Autodesk Fusion 360 part; units mm, degrees
sketch "Boceto1" plane through (0, 0, 0) normal (0, 0, 1) x (1, 0, 0)
  line L0 (-67.5, 45) -> (67.5, 45)
  line L1 (67.5, 45) -> (67.5, -45)
  line L2 (67.5, -45) -> (-67.5, -45)
  line L3 (-67.5, -45) -> (-67.5, 45)
  line L4 (-67.5, 45) -> (67.5, -45) construction
  line L5 (67.5, 45) -> (-67.5, -45) construction
  dimension "d1" = 135
  dimension "d2" = 90
extrude "Extruir1" add sketch "Boceto1" along normal blind 4
sketch "Boceto2" plane through (0, 0, 4) normal (0, 0, 1) x (-1, 0, 0)
  line L0 (67.5, 45) -> (-67.5, 45)
  line L1 (-67.5, 45) -> (-67.5, -45)
  line L2 (-67.5, -45) -> (67.5, -45)
  line L3 (67.5, -45) -> (67.5, 45)
  line L4 (67.5, -45) -> (67.5, -40)
  line L5 (67.5, -40) -> (62.5, -40)
  line L6 (67.5, 45) -> (62.5, 45)
  line L7 (62.5, 45) -> (62.5, 40)
  line L8 (-67.5, -45) -> (-62.5, -45)
  line L9 (-62.5, -45) -> (-62.5, -40)
  line L10 (-67.5, 45) -> (-67.5, 40)
  line L11 (-67.5, 40) -> (-62.5, 40)
  circle A0 centre (62.5, -40) radius 2
  circle A1 centre (62.5, 40) radius 2
  circle A2 centre (-62.5, -40) radius 2
  circle A3 centre (-62.5, 40) radius 2
  dimension "d5" = 5
  dimension "d6" = 5
  dimension "d7" = 135
  dimension "d8" = 90
  dimension "d9" = 5
  dimension "d10" = 5
  dimension "d11" = 5
  dimension "d12" = 5
  dimension "d13" = 5
  dimension "d14" = 5
  dimension "d15" = 4
  dimension "d16" = 4
  dimension "d17" = 4
  dimension "d18" = 4
extrude "Extruir2" cut sketch "Boceto2" against normal blind 4 contours A1 | A3 | A2 | A0
fillet "Empalme1" radius 5 4 edges at (-67.5, -45, 2) (67.5, -45, 2) (67.5, 45, 2) (-67.5, 45, 2)
sketch "Boceto3" plane through (0, 0, 4) normal (0, 0, 1) x (-1, 0, 0)
  circle A0 centre (62.5, 40) radius 2
  circle A1 centre (-62.5, -40) radius 2
  circle A2 centre (62.5, -40) radius 2
  circle A3 centre (-62.5, 40) radius 2
  arc A4 (62.5, -45) -> (67.5, -40) centre (62.5, -40) ccw
  line L0 (67.5, -40) -> (67.5, 40)
  arc A5 (67.5, 40) -> (62.5, 45) centre (62.5, 40) ccw
  line L1 (62.5, 45) -> (-62.5, 45)
  arc A6 (-62.5, 45) -> (-67.5, 40) centre (-62.5, 40) ccw
  line L2 (-67.5, 40) -> (-67.5, -40)
  arc A7 (-67.5, -40) -> (-62.5, -45) centre (-62.5, -40) ccw
  line L3 (-62.5, -45) -> (62.5, -45)
  line L4 (-67.5, 0) -> (-46, 0)
  circle A8 centre (-46, 0) radius 4
  circle A9 centre (-46, 0) radius 7
  line L5 (-46, 0) -> (-46, -7) construction
  line L6 (-46, 0) -> (-39, 0) construction
  line L7 (-46, 0) -> (-46, 7) construction
  line L8 (-46, 0) -> (-53, 0) construction
  circle A10 centre (-46, -7) radius 1.5
  circle A11 centre (-39, 0) radius 1.5
  circle A12 centre (-46, 7) radius 1.5
  circle A13 centre (-53, 0) radius 1.5
  dimension "d23" = 21.5
  dimension "d24" = 8
  dimension "d25" = 14
  dimension "d26" = 3
  dimension "d27" = 3
  dimension "d28" = 3
  dimension "d29" = 3
extrude "Extruir3" cut sketch "Boceto3" against normal blind 4 contours L4 A9 A13 | L4 A9 A13 | L4 A9 A13 | L4 A9 A13 | A8 | A9 A12 | A9 A12 | A9 A10 | A9 A10 | A9 A11 | A9 A11
mirror "Simetría1" about plane through (0, 0, 0) normal (1, 0, 0) of "Extruir3"
sketch "Boceto4" plane through (0, 0, 4) normal (0, 0, 1) x (-1, 0, 0)
  circle A0 centre (46, 7) radius 1.5
  circle A1 centre (46, -7) radius 1.5
  circle A2 centre (39, 0) radius 1.5
  circle A3 centre (53, 0) radius 1.5
  circle A4 centre (46, 0) radius 4
  arc A5 (62.5, -45) -> (67.5, -40) centre (62.5, -40) ccw
  line L0 (67.5, -40) -> (67.5, 40)
  arc A6 (67.5, 40) -> (62.5, 45) centre (62.5, 40) ccw
  line L1 (62.5, 45) -> (-62.5, 45)
  arc A7 (-62.5, 45) -> (-67.5, 40) centre (-62.5, 40) ccw
  line L2 (-67.5, 40) -> (-67.5, -40)
  arc A8 (-67.5, -40) -> (-62.5, -45) centre (-62.5, -40) ccw
  line L3 (-62.5, -45) -> (62.5, -45)
  circle A9 centre (-62.5, 40) radius 2
  circle A10 centre (62.5, -40) radius 2
  circle A11 centre (-62.5, -40) radius 2
  circle A12 centre (62.5, 40) radius 2
  circle A13 centre (-46, 7) radius 1.5
  circle A14 centre (-46, -7) radius 1.5
  circle A15 centre (-53, 0) radius 1.5
  circle A16 centre (-39, 0) radius 1.5
  circle A17 centre (-46, 0) radius 4
  line L4 (0, 35) -> (0, -35)
  line L5 (-20, -35) -> (20, -35)
  line L6 (-20, 35) -> (20, 35)
  line L7 (20, -30) -> (-20, -30)
  arc A18 (-20, -30) -> (-20, -40) centre (-20, -35) ccw
  line L8 (-20, -40) -> (20, -40)
  arc A19 (20, -40) -> (20, -30) centre (20, -35) ccw
  line L9 (20, -35) -> (-20, -35) construction
  line L10 (20, 40) -> (-20, 40)
  arc A20 (-20, 40) -> (-20, 30) centre (-20, 35) ccw
  line L11 (-20, 30) -> (20, 30)
  arc A21 (20, 30) -> (20, 40) centre (20, 35) ccw
  line L12 (20, 35) -> (-20, 35) construction
  dimension "d34" = 70
  dimension "d35" = 40
  dimension "d36" = 40
  dimension "d37" = 10
  dimension "d38" = 10
extrude "Extruir4" cut sketch "Boceto4" against normal blind 4 contours L7 A18 L8 A19 | L10 A20 L11 A21
Could you check a few things on this model? Use its own coordinates, in mm. Give positions to 0.01 mm unless a question says otherwise; leave off trailing zeros. Order: outer loops, then holes, each group sorted by start corner. A loop starts at its lowest first (then second) coordinate and runs counter-clockwise, first axis right, second up.
Q1. Suppose I cut it at D-D, the plane z = 3.15. Count the separate pieces of the cut face and the enclosed holes in it, and give its area (3 significant figures).
Q2. We'd pull the mould along Y, two halves only. Please class faces 1 (the cylindrical face through (54.2, 0.9, 2)), 2 (the flat face through (-1, 1, 0)), 3 (the cylindrical face through (25, -35, 2)), 4 (the cylindrical face through (66.07, 43.5, 2.03)): +Y half, -Y half, draft (parallel to the pull), parting line (faces both ways), or undercut.
Q3. Suppose I cut it at A-A, the plane x = -46. Write out the boundary of the cut face in (y, z).
Q4. Suppose I cut it at B-B, the plane x = 39. Write out the boundary of the cut face in (y, z), and give its area (3 significant figures).
Q5. If I drill on line 1 along Y through (x, z) = (3, 0.3); line 2 along Y through (x, z) = (-62.5, 2.1); line 3 along Y through (x, z) = (46, 1.1), over which ranges is the centre line in solid material (lowest first)?
Q6. Suppose I cut it at C-C, the plane y = 35. Write out the boundary of the cut face in (x, z).
Solution:
1. separate pieces: 1
1. enclosed holes: 16
1. area: 11,000 mm2
2. face 1: undercut
2. face 2: draft
2. face 3: undercut
2. face 4: +Y half
3. outline: (-45, 0) - (-8.5, 0) - (-8.5, 4) - (-45, 4) - close; (-5.5, 0) - (-4, 0) - (-4, 4) - (-5.5, 4) - close; (4, 0) - (5.5, 0) - (5.5, 4) - (4, 4) - close; (8.5, 0) - (45, 0) - (45, 4) - (8.5, 4) - close
4. outline: (-45, 0) - (-1.5, 0) - (-1.5, 4) - (-45, 4) - close; (1.5, 0) - (45, 0) - (45, 4) - (1.5, 4) - close
4. area: 348 mm2
5. line 1: y = -45 to -40, -30 to 30, 40 to 45
5. line 2: y = -45 to -42, -38 to 38, 42 to 45
5. line 3: y = -45 to -8.5, -5.5 to -4, 4 to 5.5, 8.5 to 45
6. outline: (-67.5, 0) - (-25, 0) - (-25, 4) - (-67.5, 4) - close; (25, 0) - (67.5, 0) - (67.5, 4) - (25, 4) - close
